For this review, take the finished solid that the model builds, in its own axes (mm). A direction names the side the tool comes from. Coordinates: 2 decimals unless noted, no trailing zeros. One line per question, with ' | ' between items.
from build123d import *

# Parameters (mm, degrees)
F0_W     = 1570.090592
F0_H     = 280.429076
F0_W_2   = 103.658766
F0_H_2   = 4.515674
F0_W_3   = 11.288195
F0_H_3   = 1.529689
F0_W_4   = 0.172824
F0_H_4   = 1.568052
F0_W_5   = 11.857286
F0_H_5   = 1.361676
F0_W_6   = 14.053285
F0_H_6   = 0.829553
F0_W_7   = 12.576282
F0_H_7   = 2.731625
F0_W_8   = 144.339084
F0_H_8   = 4.521026
F1_DEPTH = 25


with BuildPart() as f1:
    # F0 (on Top) → F1 (new body)
    with BuildSketch(Plane.XY):
        with Locations((-341.946453, 102.304155)):
            Rectangle(F0_W, F0_H)
        with Locations((3.491953, 30.238768)):
            Rectangle(F0_W_2, F0_H_2, mode=Mode.SUBTRACT)
        Polygon((114.178963, 3.437468), (-5.49449, 3.437468), (-5.49449, 7.963303), (114.178963, 7.963303), (167.111993, 7.963303), (179.547533, 7.963303), (179.547533, 9.387144), (234.135687, 9.387144), (234.135687, 4.629135), (233.852416, 4.629135), (233.852416, 3.437468), (167.111993, 3.437468), align=None, mode=Mode.SUBTRACT)
        with Locations((132.608905, 10.247366)):
            Rectangle(F0_W_3, F0_H_3, mode=Mode.SUBTRACT)
        with Locations((150.00771, 11.890458)):
            Rectangle(F0_W_4, F0_H_4, mode=Mode.SUBTRACT)
        with Locations((168.930627, 11.907446)):
            Rectangle(F0_W_5, F0_H_5, mode=Mode.SUBTRACT)
        with Locations((154.621362, 15.909721)):
            Rectangle(F0_W_6, F0_H_6, mode=Mode.SUBTRACT)
        with Locations((399.00133, 10.414176)):
            Rectangle(F0_W_7, F0_H_7, mode=Mode.SUBTRACT)
        with Locations((254.24999, 22.304791)):
            Rectangle(F0_W_8, F0_H_8, mode=Mode.SUBTRACT)
    extrude(amount=F1_DEPTH)


solid = f1.part
1. Machinability: for faces 1 (the flat face through (116, 3.437, 12)), 2 (the flat face through (-353, 242.519, 12)), which of the approach directions +Z, -Z, +X, -X, +Y, -Y give a long, thin tool a straight path to every point of the face, cutting with its end or side? Answer none if there is none.
Computed values:
face 1: +Z, -Z | face 2: +Z, -Z, +X, -X, +Y
2. Draft analysis for pull direction X (two halves, no side actions). For faces 3 (the flat face through (-1126.992, 100, 12)), 4 (the flat face through (86, 7.963, 12)), 5 (the flat face through (-353, 104, 25)), state which applies: pulls with the +X half, pulls with the -X half, needs draft (parallel to the pull), parting line crosses it, or undercut.
Computed values:
face 3: pulls with the -X half | face 4: undercut | face 5: needs draft
3. For line 1 along Y through (x, z) = (133, 3); line 2 along Y through (x, z) = (65, 6.5); line 3 along Y through (x, z) = (324.5, 17.5), list the stretches that pass through material, from the lowest coordinate up.
Computed values:
line 1: y = -37.91 to 3.44, 7.96 to 9.48, 11.01 to 242.52 | line 2: y = -37.91 to 3.44, 7.96 to 242.52 | line 3: y = -37.91 to 20.04, 24.57 to 242.52
